For this review, take the finished solid that the model builds, in its own axes (mm). Coordinates: 2 decimals unless noted, no trailing zeros. Order: outer loops, then holes, each group sorted by start corner. A loop starts at its lowest first (then second) coordinate and runs counter-clockwise, first axis right, second up.
from build123d import *

# Parameters (mm, degrees)
F0_W     = 88.341098
F0_H     = 38.66888
F1_DEPTH = 3.175
F2_W     = 22.6314
F2_H     = 6.916385
F3_DEPTH = 3.175
F4_W     = 22.6314
F4_H     = 6.602003
F5_DEPTH = 3.175


with BuildPart() as f1:
    # F0 (on Top) → F1 (new body)
    with BuildSketch(Plane.XY):
        with Locations((0.943141, 1.729096)):
            Rectangle(F0_W, F0_H)
    extrude(amount=F1_DEPTH)

    # F2 (on face) → F3 (join)
    with BuildSketch(Plane.XY.offset(3.175)):
        with Locations((-54.543108, 17.605344)):
            Rectangle(F2_W, F2_H)
    extrude(amount=-F3_DEPTH)

    # F4 (on face) → F5 (join)
    with BuildSketch(Plane.XY.offset(3.175)):
        with Locations((-54.543108, -14.304342)):
            Rectangle(F4_W, F4_H)
    extrude(amount=-F5_DEPTH)


solid = f1.part
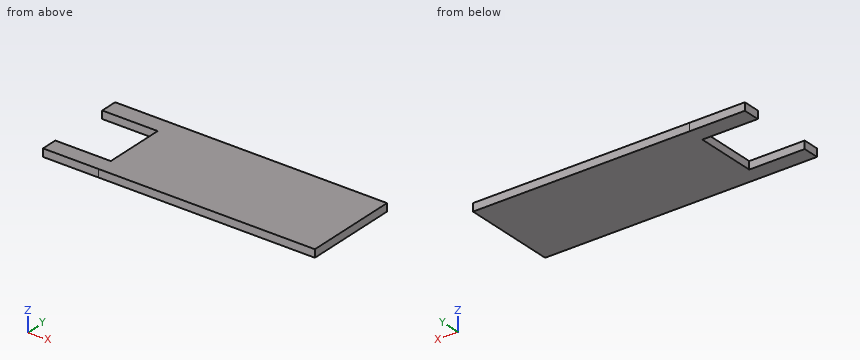
1. Clearance check with a flat-ended pin moving along its axis: pin 1 Ø1 at (y, z) = (-2.5, 2) entering from -X. State where the tip first meets the part, or that it passes through.
Answer below:
pin 1: stops at x = -43.23
2. Take a section at C-C, the plane y = 3. Give the boundary of the cut face in (x, z) (3 decimals).
Answer below:
outline: (-43.227, 0) - (45.114, 0) - (45.114, 3.175) - (-43.227, 3.175) - close
3. To check wall thickness, follow L1, parallel to Y at x = -60.5, z = 0.6; L2, parallel to X at y = 9, z = 1.2. State the ranges of each line that lie inside material, in increasing order.
Answer below:
L1: y = -17.61 to -11, 14.15 to 21.06
L2: x = -43.23 to 45.11
4. Take a section at B-B, the plane z = 0.9. Give the boundary of the cut face in (x, y).
Answer below:
outline: (-65.86, -17.61) - (45.11, -17.61) - (45.11, 21.06) - (-65.86, 21.06) - (-65.86, 14.15) - (-43.23, 14.15) - (-43.23, -11) - (-65.86, -11) - close
5. Take a section at A-A, the plane x = -50.5. Give the boundary of the cut face in (y, z) (3 decimals), plus the area to 3 significant figures.
Answer below:
outline: (-17.605, 0) - (-11.003, 0) - (-11.003, 3.175) - (-17.605, 3.175) - close; (14.147, 0) - (21.064, 0) - (21.064, 3.175) - (14.147, 3.175) - close
area: 42.9 mm2
